from build123d import *

# Parameters (mm, degrees)
F0_R            = 34.0451530949
F0_R_2          = 1.25
F0_R_3          = 7.875
F1_DEPTH        = 4.15
F3_DEPTH        = 1.25
F3_COPIES_COUNT = 4


# Not quite as in the source:
# - a pattern or mirror of a feature is missing from the dataset's text; its kind, count and spacing are read off the source's solid


with BuildPart() as f1:
    # F0 (on Top) → F1 (new body, symmetric)
    with BuildSketch(Plane.XY):
        Circle(F0_R)
        with Locations((10.6066017178, -10.6066017178)):
            Circle(F0_R_2, mode=Mode.SUBTRACT)
        Circle(F0_R_3, mode=Mode.SUBTRACT)
        with Locations((15, 0)):
            Circle(F0_R_2, mode=Mode.SUBTRACT)
        with Locations((10.6066017178, 10.6066017178)):
            Circle(F0_R_2, mode=Mode.SUBTRACT)
        with Locations((10.6066017178, 10.6066017178)):
            Circle(F0_R_2)
        with Locations((15, 0)):
            Circle(F0_R_2)
        with Locations((10.6066017178, -10.6066017178)):
            Circle(F0_R_2)
    extrude(amount=F1_DEPTH, both=True)

    # F2 (on Top) → F3 (cut, symmetric)
    with BuildSketch(Plane.XY):
        with BuildLine():
            Line((9.4432745967, 10.1492506389), (13.2777855897, 0.3957137164))
            ThreePointArc((13.2777855897, 0.3957137164), (13.3159783656, 0.3022787926), (13.3566720831, 0.2099056662))
            Line((13.3566720831, 0.2099056662), (6.3440025672, -6.039136155))
            ThreePointArc((6.3440025672, -6.039136155), (6.6944330225, -11.915202943), (12.3288161281, -10.2108880014))
            Line((12.3288161281, -10.2108880014), (15.6329589882, -1.8064058021))
            ThreePointArc((15.6329589882, -1.8064058021), (20.0264439119, -0.0879066383), (19.2625991506, 4.5674655628))
            Line((19.2625991506, 4.5674655628), (11.4382124503, 11.5398345877))
            ThreePointArc((11.4382124503, 11.5398345877), (9.891801137, 11.6320577772), (9.4432745967, 10.1492506389))
        make_face()
        with BuildLine():
            ThreePointArc((10.0021618859, -9.2961858437), (8.1240341841, -9.8642908242), (8.0072240323, -7.9056018949))
            Line((8.0072240323, -7.9056018949), (11.9194173824, -4.4194173824))
            Line((11.9194173824, -4.4194173824), (10.0021618859, -9.2961858437))
        make_face(mode=Mode.SUBTRACT)
        with BuildLine():
            ThreePointArc((17.5993776855, 2.7009998229), (17.4825675337, 0.7423108936), (15.6044398319, 1.3104158741))
            Line((15.6044398319, 1.3104158741), (13.6871843354, 6.1871843354))
            Line((13.6871843354, 6.1871843354), (17.5993776855, 2.7009998229))
        make_face(mode=Mode.SUBTRACT)
    f3 = extrude(amount=F3_DEPTH, both=True, mode=Mode.SUBTRACT)

    # F3_copies: F3 ×4 about axis
    f3_copies_axis = Axis((0, 0, 0), (0, 0, 1))
    for i in range(1, F3_COPIES_COUNT):
        add(f3.rotate(f3_copies_axis, i * 360 / F3_COPIES_COUNT), mode=Mode.SUBTRACT)


solid = f1.part
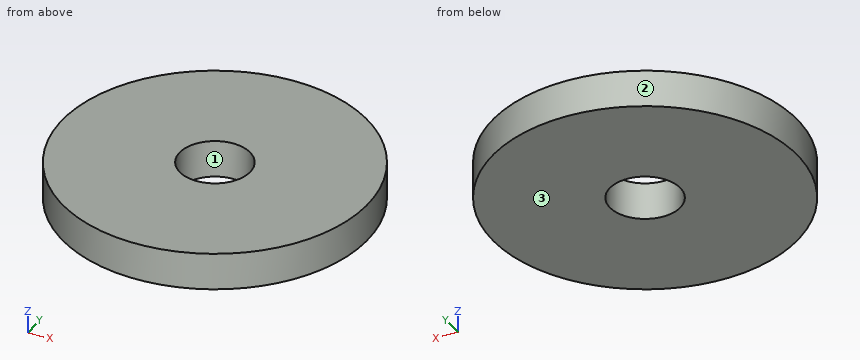
The listing builds one solid part. Answer for the finished solid, in the listing's coordinates (mm). Face numbers are marked on the shaded views. Round coordinates to 2 decimals unless told otherwise and drop trailing zeros. Write each loop counter-clockwise with the first axis right and the second up, starting at its lowest first coordinate (ties: lowest second). Pieces come first, ordered by that corner, then holes. Notation, with made-up numbers: M -5,8 L 29,8 A23 ccw 29,36 Z; hole C 67.25,-29.5 d9. An arc over 180 degrees is marked long. Write each question's results on one line, items separated by ' | '. Start each with the question number.
(1) The part is cut by section A-A, the plane z = 0. Give the number of separate pieces and of enclosed holes in the cut face, and give its area (3 significant figures).
(2) Determine the mould class of the marked faces 1, 2 and 3 for opening direction Y: +Y half, -Y half, draft (parallel to the pull), parting line (faces both ways), or undercut.
(3) Each of these flat-tipped pins is pushed along its axis until it touches: P1, Ø1.5, axis at x = -7.5, z = -1, coming from the +Y side; P2, Ø3, axis at x = 2.5, z = -2.5, coming from the -Y side; P3, Ø10, axis at x = 1, y = -2.5, coming from the +Z side; P4, Ø3, axis at y = -23, z = -2.5, coming from the -X side. Where does it stop, or does it pass through?
(4) Find the intervals of material crossed by line 1 (Y direction, x = 17, z = 0); line 2 (Z direction, x = 18.5, y = 0.5); line 3 (Y direction, x = 0, z = 1) (3 decimals), in increasing order.
(5) The part is cut by section B-B, the plane y = -22.5. Write down the section's boundary in (x, z), and give its area (3 significant figures).
Worked answers:
1) separate pieces: 10 | enclosed holes: 2 | area: 2,950 mm²
2) face 1: undercut | face 2: parting line | face 3: draft
3) P1: stops at y = 33.37 | P2: stops at y = -34.03 | P3: passes through | P4: stops at x = -26.4
4) line 1: y = -29.5 to -1.98, 0.54 to 3.24, 6.58 to 29.5 | line 2: z = -4.15 to -1.25, 1.25 to 4.15 | line 3: y = -34.045 to -20.075, -13.121 to -7.875, 7.875 to 13.121, 20.075 to 34.045
5) outline: M -25.55,-4.15 L 25.55,-4.15 L 25.55,4.15 L -25.55,4.15 Z | area: 424 mm²
